Part model, mm, in its own coordinate system. A direction names the side the tool comes from. Give positions to 0.01 mm unless a question says otherwise; leave off trailing zeros. Order: outer loops, then holes, each group sorted by start corner. A loop starts at its lowest first (then second) coordinate and runs counter-clockwise, first axis right, second up. Notation, with made-up numbers: (50.25, 34) - (106.25, 34) arc R12 cw to (106.25, 57) - close; hole circle Ø1 at (33.25, 77.25). An arc over 180 degrees is marked (long way). One line per item, written item: value.
```python
from build123d import *
from OCP.BRepFilletAPI import BRepFilletAPI_MakeChamfer

# Parameters (mm, degrees)
BOSS_EXTRUDE2_DEPTH     = 38.1
CHAMFER2_SIZE           = 38.1
CHAMFER2_SIZE_2         = 25.4
SKETCH6_W               = 9.525
SKETCH6_H               = 12.7
CUT_EXTRUDE3_DEPTH      = 206.929041238
SKETCH7_R               = 10.9855
SKETCH7_R_2             = 1.8415
CUT_EXTRUDE4_DEPTH      = 207.992468583
SKETCH8_W               = 69.85
SKETCH8_H               = 45.790501198
BOSS_EXTRUDE3_DEPTH     = 6.35
CUT_EXTRUDE5_DEPTH      = 208.669669805
CUT_EXTRUDE5_DEPTH_BACK = 208.669669805
BOSS_EXTRUDE4_DEPTH     = 69.85
BOSS_EXTRUDE5_DEPTH     = 69.85
SKETCH12_R              = 1.8288
CUT_EXTRUDE6_DEPTH      = 210.393754689
SKETCH13_R              = 1.8288
CUT_EXTRUDE7_DEPTH      = 12.7
FILLET1_R               = 3.175


with BuildPart() as part:
    # Sketch4 → Boss-Extrude2 (new body)
    with BuildSketch(Plane(origin=(0, 0, 0), x_dir=(1, 0, 0), z_dir=(0, 1, 0))):
        with BuildLine():
            Line((0, 0), (0, -54.242759604))
            ThreePointArc((0, -54.242759604), (-1.905, -58.208333333), (0, -62.173907062))
            Line((0, -62.173907062), (0, -107.159426271))
            ThreePointArc((0, -107.159426271), (-0.417102448, -114.717102448), (7.140573729, -114.3))
            Line((7.140573729, -114.3), (52.126092938, -114.3))
            ThreePointArc((52.126092938, -114.3), (56.091666667, -116.205), (60.057240396, -114.3))
            Line((60.057240396, -114.3), (105.042759604, -114.3))
            ThreePointArc((105.042759604, -114.3), (109.008333333, -116.205), (112.973907062, -114.3))
            Line((112.973907062, -114.3), (157.959426271, -114.3))
            ThreePointArc((157.959426271, -114.3), (165.517102448, -114.717102448), (165.1, -107.159426271))
            Line((165.1, -107.159426271), (165.1, -62.173907062))
            ThreePointArc((165.1, -62.173907062), (167.005, -58.208333333), (165.1, -54.242759604))
            Line((165.1, -54.242759604), (165.1, 0))
            Line((165.1, 0), (158.75, 0))
            Line((158.75, 0), (158.75, -54.242759604))
            ThreePointArc((158.75, -54.242759604), (156.845, -58.208333333), (158.75, -62.173907062))
            Line((158.75, -62.173907062), (158.75, -107.159426271))
            ThreePointArc((158.75, -107.159426271), (158.332897552, -107.532897552), (157.959426271, -107.95))
            Line((157.959426271, -107.95), (112.973907062, -107.95))
            ThreePointArc((112.973907062, -107.95), (109.008333333, -106.045), (105.042759604, -107.95))
            Line((105.042759604, -107.95), (60.057240396, -107.95))
            ThreePointArc((60.057240396, -107.95), (56.091666667, -106.045), (52.126092938, -107.95))
            Line((52.126092938, -107.95), (7.140573729, -107.95))
            ThreePointArc((7.140573729, -107.95), (6.767102448, -107.532897552), (6.35, -107.159426271))
            Line((6.35, -107.159426271), (6.35, -62.173907062))
            ThreePointArc((6.35, -62.173907062), (8.255, -58.208333333), (6.35, -54.242759604))
            Line((6.35, -54.242759604), (6.35, 0))
            Line((6.35, 0), (0, 0))
        make_face()
        Polygon((0, -56.375246229), (0, -60.041420438), (3.175, -61.874507543), (6.35, -60.041420438), (6.35, -56.375246229), (3.175, -54.542159124), align=None, mode=Mode.SUBTRACT)
        Polygon((3.175, -107.458825791), (0, -109.291912895), (0, -112.958087105), (3.175, -114.791174209), (6.35, -112.958087105), (6.35, -109.291912895), align=None, mode=Mode.SUBTRACT)
        Polygon((56.091666667, -107.458825791), (52.916666667, -109.291912895), (52.916666667, -112.958087105), (56.091666667, -114.791174209), (59.266666667, -112.958087105), (59.266666667, -109.291912895), align=None, mode=Mode.SUBTRACT)
        Polygon((109.008333333, -107.458825791), (105.833333333, -109.291912895), (105.833333333, -112.958087105), (109.008333333, -114.791174209), (112.183333333, -112.958087105), (112.183333333, -109.291912895), align=None, mode=Mode.SUBTRACT)
        Polygon((161.925, -107.458825791), (158.75, -109.291912895), (158.75, -112.958087105), (161.925, -114.791174209), (165.1, -112.958087105), (165.1, -109.291912895), align=None, mode=Mode.SUBTRACT)
        Polygon((161.925, -54.542159124), (158.75, -56.375246229), (158.75, -60.041420438), (161.925, -61.874507543), (165.1, -60.041420438), (165.1, -56.375246229), align=None, mode=Mode.SUBTRACT)
    extrude(amount=BOSS_EXTRUDE2_DEPTH)

    # Chamfer2
    chamfer2_edges_1 = [part.edges().sort_by_distance(p)[0] for p in [
        (161.925, 38.1, 0),
    ]]
    chamfer2_side_1 = [part.faces().sort_by_distance(p)[0] for p in [
        (161.925, 37.592, 0),
    ]]
    chamfer2_edges_2 = [part.edges().sort_by_distance(p)[0] for p in [
        (3.175, 38.1, 0),
    ]]
    chamfer2_side_2 = [part.faces().sort_by_distance(p)[0] for p in [
        (3.175, 37.592, 0),
    ]]
    chamfer2 = BRepFilletAPI_MakeChamfer(part.part.solid().wrapped)
    for e in chamfer2_edges_1:
        chamfer2.Add(CHAMFER2_SIZE - 0.0001, CHAMFER2_SIZE_2 - 0.0001, e.wrapped, chamfer2_side_1[0].wrapped)
    for e in chamfer2_edges_2:
        chamfer2.Add(CHAMFER2_SIZE - 0.0001, CHAMFER2_SIZE_2 - 0.0001, e.wrapped, chamfer2_side_2[0].wrapped)
    add(Compound.cast(chamfer2.Shape()), mode=Mode.REPLACE)  # a hair under: the kernel refuses the full size

    # Sketch6 → Cut-Extrude3 (cut, through all)
    with BuildSketch(Plane.XY.offset(114.3)):
        with Locations((65.0875, 31.75)):
            Rectangle(SKETCH6_W, SKETCH6_H)
        with Locations((100.0125, 31.75)):
            Rectangle(SKETCH6_W, SKETCH6_H)
    extrude(amount=-CUT_EXTRUDE3_DEPTH, mode=Mode.SUBTRACT)

    # Sketch7 → Cut-Extrude4 (cut, through all)
    with BuildSketch(Plane(origin=(165.1, 0, 0), x_dir=(0, 0, -1), z_dir=(1, 0, 0))):
        with Locations((-84.666666667, 19.05)):
            Circle(SKETCH7_R)
        with Locations((-71.666666667, 32.05)):
            Circle(SKETCH7_R_2)
        with Locations((-71.666666667, 6.05)):
            Circle(SKETCH7_R_2)
        with Locations((-97.666666667, 6.05)):
            Circle(SKETCH7_R_2)
        with Locations((-97.666666667, 32.05)):
            Circle(SKETCH7_R_2)
    extrude(amount=-CUT_EXTRUDE4_DEPTH, mode=Mode.SUBTRACT)

    # Sketch8 → Boss-Extrude3 (add)
    with BuildSketch(Plane(origin=(0, 0, 0), x_dir=(-1, 0, 0), z_dir=(0, 0.5547001962252279, -0.8320502943378446))):
        with Locations((-130.175, 22.895250599)):
            Rectangle(SKETCH8_W, SKETCH8_H)
        with Locations((-34.925, 22.895250599)):
            Rectangle(SKETCH8_W, SKETCH8_H)
    extrude(amount=BOSS_EXTRUDE3_DEPTH)

    # Sketch9 → Cut-Extrude5 (cut, two sides: drawn at the far end of the back side and taken through both)
    with BuildSketch(Plane(origin=(165.1, 0, 0), x_dir=(0, 0, -1), z_dir=(1, 0, 0)).offset(-CUT_EXTRUDE5_DEPTH_BACK)):
        Polygon((-25.4, 38.1), (-17.7682498, 38.1), (-20.116480631, 41.622346246), align=None)
    extrude(amount=CUT_EXTRUDE5_DEPTH + CUT_EXTRUDE5_DEPTH_BACK, mode=Mode.SUBTRACT)

    # Sketch10 → Boss-Extrude4 (add)
    with BuildSketch(Plane(origin=(165.1, 0, 0), x_dir=(0, 0, -1), z_dir=(1, 0, 0))):
        Polygon((0, 0), (7.6317502, 0), (5.283519369, 3.522346246), align=None)
    extrude(amount=-BOSS_EXTRUDE4_DEPTH)

    # Sketch11 → Boss-Extrude5 (add)
    with BuildSketch(Plane.ZY):
        Polygon((-5.283519369, 3.522346246), (-7.6317502, 0), (0, 0), align=None)
    extrude(amount=-BOSS_EXTRUDE5_DEPTH)

    # Sketch12 → Cut-Extrude6 (cut, through all)
    with BuildSketch(Plane(origin=(0, 3.522346246, -5.283519369), x_dir=(-1, 0, 0), z_dir=(0, 0.5547001962252279, -0.8320502943378446))):
        with Locations(Location((-65.0875, 35.207167865, 0), (0, 0, 90))):
            Circle(SKETCH12_R)
        with Locations(Location((-65.0875, 2.116666667, 0), (0, 0, 90))):
            Circle(SKETCH12_R)
        with Locations(Location((-100.0125, 35.207167865, 0), (0, 0, 90))):
            Circle(SKETCH12_R)
        with Locations(Location((-100.0125, 2.116666667, 0), (0, 0, 90))):
            Circle(SKETCH12_R)
    extrude(amount=-CUT_EXTRUDE6_DEPTH, mode=Mode.SUBTRACT)

    # Sketch13 → Cut-Extrude7 (cut)
    with BuildSketch(Plane(origin=(0, 3.522346246, -5.283519369), x_dir=(-1, 0, 0), z_dir=(0, 0.5547001962252279, -0.8320502943378446))):
        with Locations(Location((-161.925, 35.207167865, 0), (0, 0, 90))):
            Circle(SKETCH13_R)
        with Locations(Location((-161.925, 18.661917266, 0), (0, 0, 90))):
            Circle(SKETCH13_R)
        with Locations(Location((-100.0125, 18.661917266, 0), (0, 0, 90))):
            Circle(SKETCH13_R)
        with Locations(Location((-3.175, 18.661917266, 0), (0, 0, 270))):
            Circle(SKETCH13_R)
        with Locations(Location((-3.175, 35.207167865, 0), (0, 0, 270))):
            Circle(SKETCH13_R)
        with Locations(Location((-65.0875, 18.661917266, 0), (0, 0, 270))):
            Circle(SKETCH13_R)
    extrude(amount=-CUT_EXTRUDE7_DEPTH, mode=Mode.SUBTRACT)

    # Fillet1
    fillet1_edges = [part.edges().sort_by_distance(p)[0] for p in [
        (100.0125, 25.4, 107.95),
        (65.0875, 25.4, 107.95),
        (127, 38.1, 25.4),
        (38.1, 38.1, 25.4),
    ]]
    fillet(fillet1_edges, radius=FILLET1_R)


solid = part.part
```
1) Pin check, flat tips, straight feed: pin 1 (1 mm diameter, centred on x = 128.5, y = 26.5, fed in from -Z); pin 2 (5 mm diameter, centred on y = 13.5, z = 67.5, fed in from +X); pin 3 (5 mm diameter, centred on x = 89.5, y = 26, fed in from +Z); pin 4 (3.5 mm diameter, centred on y = 6.05, z = 71.67, fed in from +X). Stop position of each tip, or through.
Outcome:
pin 1: stops at z = 9.7
pin 2: stops at x = 165.1
pin 3: stops at z = 114.3
pin 4: passes through
2) Which spindle directions (+Z, -Z, +X, -X, +Y, -Y) get a long thin tool onto all of the face, cutting with end or side? Do faces 4 (the flat face through (165.1, 19, 31)), 5 (the flat face through (105.833, 19, 111)), 6 (the flat face through (38.5, 16.8, 11.2)). Say none if no direction does.
Outcome:
face 4: -Z, +X, +Y, -Y
face 5: +Y, -Y
face 6: -Y
3) Cut at B-B, the plane z = 82. Give the cut face in (x, y).
Outcome:
outline: (0, 0) - (6.35, 0) - (6.35, 8.39) - (0, 8.39) - close; (0, 29.71) - (6.35, 29.71) - (6.35, 38.1) - (0, 38.1) - close; (158.75, 0) - (165.1, 0) - (165.1, 8.39) - (158.75, 8.39) - close; (158.75, 29.71) - (165.1, 29.71) - (165.1, 38.1) - (158.75, 38.1) - close
4) Cut at A-A, the plane z = 39. Give the cut face in (x, y), then the cut area to 3 significant figures.
Outcome:
outline: (0, 0) - (6.35, 0) - (6.35, 38.1) - (0, 38.1) - close; (158.75, 0) - (165.1, 0) - (165.1, 38.1) - (158.75, 38.1) - close
area: 484 mm^2
5) Drill centre lines: line 1 along Z through (x, y) = (161, 6); line 2 along X through (y, z) = (13.5, 105). Where is each one in solid material? Low to high. Write a range as from..to.
Outcome:
line 1: z = -3.63..55.08, 61.34..69.83, 73.51..95.83, 99.51..107.99, 114.26..116.12
line 2: x = 0..6.35, 158.75..165.1
6) Mould opens along X. For faces 1 (the flat face through (95.25, 19, 8)), 2 (the flat face through (165.1, 14.5, 95)), 3 (the flat face through (160, 38.1, 70)) say: released by +X, released by -X, zero draft, split by the parting line, or undercut.
Outcome:
face 1: undercut
face 2: released by +X
face 3: zero draft
